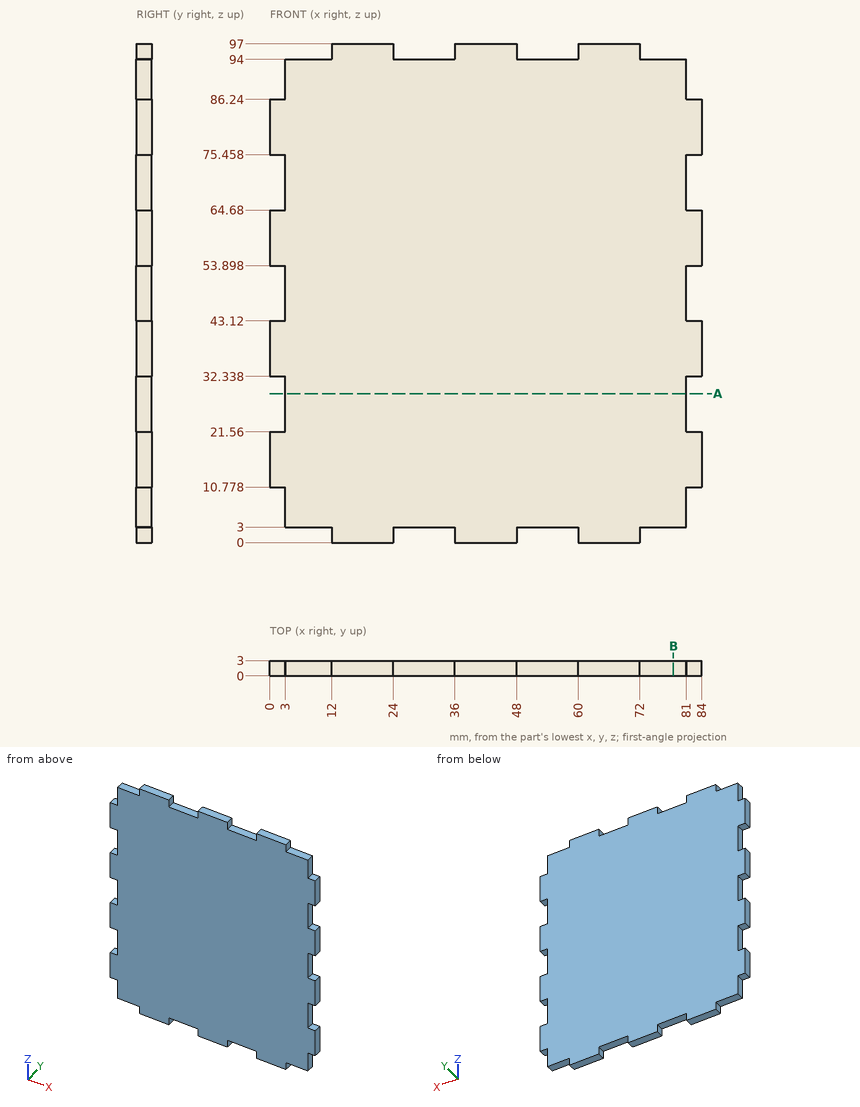
Source: three-view drawing plus pictorial views. Frame: mm from the lowest corner of the part. Give positions to 0.01 mm unless a question says otherwise; leave off trailing zeros. Write each loop counter-clockwise with the first axis right and the second up, starting at its lowest first coordinate (ties: lowest second). Pieces come first, ordered by that corner, then holes. Notation, with made-up numbers: (82, -40) -> (118, -40) arc R18 ccw to (118, -9) -> close; hole circle Ø2 at (-9, -16). An arc over 180 degrees is marked (long way). Answer in a Markdown table with one row per item.
(1) Ray query, line 1 along Z through (x, y) = (73.5, 1); line 2 along X through (y, z) = (2.8, 22.5). Return the intervals inside material, ascending. Write a range as [from, to].
Answers below:
| item | result |
|---|---|
| line 1 | [3, 94] |
| line 2 | [3, 81] |
(2) Pin query (flat end, axial travel): pin 1 (0.9 mm diameter, centred on y = 1.5, z = 5, fed in from -X); pin 2 (1.5 mm diameter, centred on x = 82.5, y = 2, fed in from -Z); pin 3 (0.9 mm diameter, centred on x = 53, y = 2, fed in from -Z). Return the tip coordinate at first contact, or that it passes through.
Answers below:
| item | result |
|---|---|
| pin 1 | x = 3 |
| pin 2 | z = 10.78 |
| pin 3 | z = 3 |
(3) Section query A-A on z = 29. Return loops of the section in (x, y), then the cut area to 3 significant figures.
Answers below:
| item | result |
|---|---|
| outline | (3, 0) -> (81, 0) -> (81, 3) -> (3, 3) -> close |
| area | 234 mm^2 |
(4) Section query B-B on x = 78.5. Return loops of the section in (y, z), then the cut area to 3 significant figures.
Answers below:
| item | result |
|---|---|
| outline | (0, 3) -> (3, 3) -> (3, 94) -> (0, 94) -> close |
| area | 273 mm^2 |
